Autodesk Inventor part; units mm, degrees
ref_plane "YZ Plane" through (0, 0, 0) normal (1, 0, 0) x (0, 1, 0)
ref_plane "XZ Plane" through (0, 0, 0) normal (0, 1, 0) x (-1, 0, 0)
ref_plane "XY Plane" through (0, 0, 0) normal (0, 0, 1) x (1, 0, 0)
sketch "Sketch1" plane through (0, 0, 0) normal (0, 0, 1) x (1, 0, 0)
  line L0 (2.05, 2.05) -> (-2.05, 2.05)
  line L1 (-2.05, 2.05) -> (-2.05, -2.05)
  line L2 (-2.05, -2.05) -> (2.05, -2.05)
  line L3 (2.05, -2.05) -> (2.05, 2.05)
  line L4 (2.05, 2.05) -> (-2.05, -2.05) construction
  line L5 (-2.05, 2.05) -> (2.05, -2.05) construction
  line L6 (4.05, 4.05) -> (-4.05, 4.05)
  line L7 (-4.05, 4.05) -> (-4.05, -4.05)
  line L8 (-4.05, -4.05) -> (4.05, -4.05)
  line L9 (4.05, -4.05) -> (4.05, 4.05)
  line L10 (4.05, 4.05) -> (-4.05, -4.05) construction
  line L11 (-4.05, 4.05) -> (4.05, -4.05) construction
  point P0 (0, 0)
  point P1 (0, 0)
  point P2 (0, 0)
  point P3 (0, 0)
  dimension "d24" = 8.1
  dimension "d25" = 4.1
  dimension "d26" = 8.1
extrude "Extrusion1" add sketch "Sketch1" along normal blind 6.5
sketch "Sketch2" plane through (-5.0868, 4.05, 0) normal (0, 1, 0) x (1, 0, 0)
  circle A0 centre (14.0868, -3.25) radius 1.5
  circle A1 centre (-3.9132, -3.25) radius 1.5
  line L0 (12, 0) -> (0, 0)
  line L1 (12, -6.5) -> (0, -6.5)
  line L2 (-7.9132, -6.5) -> (18.0868, -6.5)
  line L3 (18.0868, -6.5) -> (18.0868, 0)
  line L4 (18.0868, 0) -> (-7.9132, 0)
  line L5 (-7.9132, 0) -> (-7.9132, -6.5)
  line L6 (5.0868, -6.5) -> (5.0868, 0) construction
  line L7 (1.0368, 0) -> (1.0368, -6.5)
  line L8 (9.1368, 0) -> (9.1368, -6.5)
  point P0 (5.0868, 0)
  dimension "d8" = 3
  dimension "d9" = 3
  dimension "d10" = 18
  dimension "d11" = 6.5
  dimension "d14" = 4
  dimension "d15" = 4
  dimension "d16" = 3.25
  dimension "d17" = 3.25
  dimension "d18" = 0
  dimension "d23" = 3.25
  dimension "d30" = 26
  dimension "d31" = 8.1
  dimension "d32" = 8.95
extrude "Extrusion2" add sketch "Sketch2" along normal blind 4
fillet "Fillet1" radius 2 2 edges at (4.05, 4.05, 3.25) (-4.05, 4.05, 3.25)
fillet "Fillet2" radius 2 2 edges at (-4.05, -4.05, 3.25) (4.05, -4.05, 3.25)
fillet "Fillet3" radius 2 4 edges at (-13, 6.05, 6.5) (13, 6.05, 6.5) (13, 6.05, 0) (-13, 6.05, 0)
sketch "Sketch3" plane through (-5.0868, 8.05, 0) normal (0, 1, 0) x (1, 0, 0)
  line L0 (-5.9132, -6.5) -> (16.0868, -6.5)
  line L1 (16.0868, 0) -> (-5.9132, 0)
  line L2 (11.0868, -6.5) -> (-0.9132, -6.5)
  line L3 (-0.9132, -6.5) -> (-0.9132, 0)
  line L4 (-0.9132, 0) -> (11.0868, 0)
  line L5 (11.0868, 0) -> (11.0868, -6.5)
  line L6 (-7.9132, -2) -> (-7.9132, -4.5)
  line L7 (18.0868, -4.5) -> (18.0868, -2)
  point P0 (5.0868, 0)
  point P1 (11.0868, 0)
  point P2 (-0.9132, -6.5)
  dimension "d33" = 7
  dimension "d34" = 7
extrude "Extrusion3" cut sketch "Sketch3" against normal blind 2
fillet "Fillet4" radius 0.5 4 edges at (6, 8.05, 3.25) (-6, 8.05, 3.25) (-6, 6.05, 3.25) (6, 6.05, 3.25)
mirror "Mirror1" about plane through (0, 0, 0) normal (0, 1, 0)
sketch "Sketch5" plane through (6.5, -8.05, 0) normal (0, -1, 0) x (1, 0, 0)
  line L0 (12.0758, -8.2102) -> (-27.8852, -8.2102)
  line L1 (-27.8852, -8.2102) -> (-27.8852, 11.7461)
  line L2 (-27.8852, 11.7461) -> (12.0758, 11.7461)
  line L3 (12.0758, 11.7461) -> (12.0758, -8.2102)
  point P0 (-6.5, 0)
extrude "Extrusion4" cut sketch "Sketch5" against normal up to surface (2 mm away)
equation "\"d16\" = d17"
equation "\"d23\" = d17"
equation "\"d32\" = -0.5 * d31 + 0.5 * d30"
properties part number "fuselage_CM904_interface" material "ABS Plastic"
Here's how the part is built. I have some questions about the finished solid (model axes, mm). A direction names the side the tool comes from. Give positions to 0.01 mm unless a question says otherwise; leave off trailing zeros. Write each loop counter-clockwise with the first axis right and the second up, starting at its lowest first coordinate (ties: lowest second). Pieces come first, ordered by that corner, then holes. Notation, with made-up numbers: M -27,10.5 L -19,10.5 A28 ccw -19,42.5 Z; hole C 65,42 d1. An arc over 180 degrees is marked long. Put each result on its own line as item: value. Start each with the question number.
Item 1: If we section it at C-C, the plane x = 9: Write out the boundary of the cut face in (y, z).
Item 2: If we section it at D-D, the plane z = 0.5: Write out the boundary of the cut face in (x, y), then the cut area to 3 significant figures.
Item 3: If we section it at B-B, the plane x = 0.25: Write out the boundary of the cut face in (y, z).
Item 4: I need wall thicknesses on L1, parallel to X at y = 5.15, z = 3.25; L2, parallel to X at y = 6.5, z = 3.25; L3, parallel to Z at x = 9, y = -5. Which ranges of each line are inside material? Lowest first, please. Write a range as from..to.
Item 5: On a 3-axis mill with a long thin cutter (end or side, diameter ignored), from which of +Z, -Z, +X, -X, +Y, -Y can I reach the whole of each face in a straight line? I mean faces 1 (the flat face through (11, 4.05, 3)), 2 (the flat face through (13, -5, 3)), 3 (the flat face through (-6, 7, 3)). Say none if no direction works.
Item 6: If we section it at A-A, the plane y = 0: Write out the boundary of the cut face in (x, z), then the cut area to 3 significant figures.
Item 7: Will these pins go through, and if not, where does the flat tip stop? pin 1 (3.5 mm diameter, centred on y = -1, z = 4, fed in from -X); pin 2 (1.8 mm diameter, centred on x = -9, z = 3.25, fed in from +Y); pin 3 (2 mm diameter, centred on y = 0.5, z = 3, fed in from +X).
Item 8: Thinking about a two-plate mould opening in Y: for faces 4 (the cylindrical face through (12.4, -5.06, 0.57)), 5 (the cylindrical face through (-4.65, -3.48, 3.3)), 6 (the cylindrical face through (-4.62, 3.45, 3.3)), 7 (the flat face through (0, 6.05, 3)), which applies, +Y half, -Y half, draft (parallel to the pull), parting line (faces both ways), or undercut?
Values:
1. outline: M -6.05,0 L -4.05,0 L -4.05,1.75 L -6.05,1.75 Z; M -6.05,4.75 L -4.05,4.75 L -4.05,6.5 L -6.05,6.5 Z; M 4.05,0 L 8.05,0 L 8.05,1.75 L 4.05,1.75 Z; M 4.05,4.75 L 8.05,4.75 L 8.05,6.5 L 4.05,6.5 Z
2. outline: M -12.32,-6.05 L 12.32,-6.05 L 12.32,-4.05 L 6.05,-4.05 A2 cw 4.05,-2.05 L 4.05,2.05 A2 cw 6.05,4.05 L 12.32,4.05 L 12.32,8.05 L 6.5,8.05 A0.5 ccw 6,7.55 L 6,6.55 A0.5 cw 5.5,6.05 L -5.5,6.05 A0.5 cw -6,6.55 L -6,7.55 A0.5 ccw -6.5,8.05 L -12.32,8.05 L -12.32,4.05 L -6.05,4.05 A2 cw -4.05,2.05 L -4.05,-2.05 A2 cw -6.05,-4.05 L -12.32,-4.05 Z; hole M -2.05,-2.05 L 2.05,-2.05 L 2.05,2.05 L -2.05,2.05 Z
2. area: 176 mm²
3. outline: M -6.05,0 L -2.05,0 L -2.05,6.5 L -6.05,6.5 Z; M 2.05,0 L 6.05,0 L 6.05,6.5 L 2.05,6.5 Z
4. L1: -13..-10.5, -7.5..7.5, 10.5..13
4. L2: -13..-10.5, -7.5..-6, 6..7.5, 10.5..13
4. L3: 0..1.75, 4.75..6.5
5. face 1: +Z, -Z, +X
5. face 2: +Z, -Z, +X, +Y, -Y
5. face 3: +Z, -Z, +Y
6. outline: M -4.05,0 L -2.05,0 L -2.05,6.5 L -4.05,6.5 Z; M 2.05,0 L 4.05,0 L 4.05,6.5 L 2.05,6.5 Z
6. area: 26.0 mm²
7. pin 1: x = -4.18
7. pin 2: through
7. pin 3: x = 4.05
8. face 4: draft
8. face 5: undercut
8. face 6: undercut
8. face 7: +Y half
